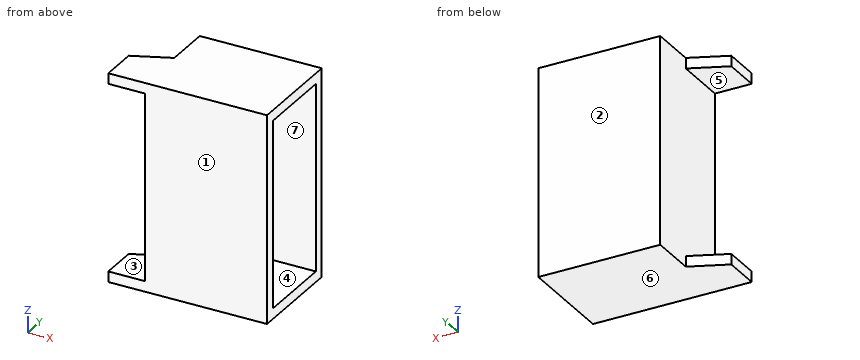
```python
from build123d import *

# Parameters (mm, degrees)
SKETCH1_W           = 5.8928
SKETCH1_H           = 10.033
BOSS_EXTRUDE1_DEPTH = 4.7625
SHELL3_T            = -0.508
BOSS_EXTRUDE2_DEPTH = 0.508
BOSS_EXTRUDE3_DEPTH = 0.508


with BuildPart() as part:
    # Sketch1 → Boss-Extrude1 (new body)
    with BuildSketch(Plane(origin=(0, 0, 0), x_dir=(1, 0, 0), z_dir=(0, 1, 0))):
        with Locations((2.9464, 5.0165)):
            Rectangle(SKETCH1_W, SKETCH1_H)
    extrude(amount=BOSS_EXTRUDE1_DEPTH)

    # Shell3
    shell3_openings = [part.faces().sort_by_distance(p)[0] for p in [
        (5.8928, 2.38125, -5.0165),
    ]]
    offset(amount=SHELL3_T, openings=shell3_openings, kind=Kind.INTERSECTION)

    # Sketch2 → Boss-Extrude2 (add)
    with BuildSketch(Plane.XY):
        Polygon((-1.778, 1.778), (0, 2.54), (0, 0), (-1.778, 0), align=None)
    extrude(amount=-BOSS_EXTRUDE2_DEPTH)

    # Sketch3 → Boss-Extrude3 (add)
    with BuildSketch(Plane(origin=(0, 0, -10.033), x_dir=(-1, 0, 0), z_dir=(0, 0, -1))):
        Polygon((0, 2.54), (1.778, 1.778), (1.778, 0), (0, 0), (0, 1.778), align=None)
    extrude(amount=-BOSS_EXTRUDE3_DEPTH)


solid = part.part
```
Here's how the part is built. I have some questions about the finished solid (model axes, mm). Face numbers are marked on the shaded views. A direction names the side the tool comes from. Coordinates: 2 decimals unless noted, no trailing zeros. Order: outer loops, then holes, each group sorted by start corner. A loop starts at its lowest first (then second) coordinate and runs counter-clockwise, first axis right, second up.
1) Imagine slicing it at A-A on z = -7. List the corners of the cut face in (x, y) for me, and give its area (3 significant figures).
2) Imagine slicing it at C-C on y = 3.5. List the corners of the cut face in (x, z) for me (3 decimals), and give its area (3 significant figures).
3) Will these pins go through, and if not, where does the flat tip stop? pin 1 (1.9 mm diameter, centred on y = 3, z = -5.5, fed in from +X); pin 2 (1.4 mm diameter, centred on y = 2, z = -3, fed in from -X).
4) Imagine slicing it at D-D on x = -1. List the corners of the cut face in (y, z) for me (3 decimals), and give its area (3 significant figures).
5) I need wall thicknesses on line 1 (Z direction, x = 5.75, y = 2.75) (3 decimals); line 2 (Y direction, x = 0.75, z = -2.5); line 3 (X direction, y = 3.75, z = -5). Which ranges of each line are inside material? Lowest first, please.
6) We'd pull the mould along Y, two halves only. Please class the marked faces 1, 2, 3 and 4: +Y half, -Y half, draft (parallel to the pull), parting line (faces both ways), or undercut.
7) Which directions (+Z, -Z, +X, -X, +Y, -Y) give clear straight access to the entire face, cutting with the end or side of a thin tool? Please do the marked faces 5, 6 and 7.
8) Imagine slicing it at B-B on x = 2. List the corners of the cut face in (y, z) for me (1 decimal), and give its area (3 significant figures).
Response values:
1. outline: (0, 0) - (5.89, 0) - (5.89, 0.51) - (0.51, 0.51) - (0.51, 4.25) - (5.89, 4.25) - (5.89, 4.76) - (0, 4.76) - close
1. area: 7.89 mm2
2. outline: (0, -10.033) - (5.893, -10.033) - (5.893, -9.525) - (0.508, -9.525) - (0.508, -0.508) - (5.893, -0.508) - (5.893, 0) - (0, 0) - close
2. area: 10.6 mm2
3. pin 1: stops at x = 0.51
3. pin 2: stops at x = 0
4. outline: (0, -10.033) - (2.111, -10.033) - (2.111, -9.525) - (0, -9.525) - close; (0, -0.508) - (2.111, -0.508) - (2.111, 0) - (0, 0) - close
4. area: 2.15 mm2
5. line 1: z = -10.033 to -9.525, -0.508 to 0
5. line 2: y = 0 to 0.51, 4.25 to 4.76
5. line 3: x = 0 to 0.51
6. face 1: -Y half
6. face 2: +Y half
6. face 3: draft
6. face 4: undercut
7. face 5: -X, +Y, -Y
7. face 6: -Z, +X, -X, +Y, -Y
7. face 7: +X
8. outline: (0, -10) - (4.8, -10) - (4.8, 0) - (0, 0) - close; hole (0.5, -9.5) - (4.3, -9.5) - (4.3, -0.5) - (0.5, -0.5) - close
8. area: 14.0 mm2
